Build history of the part. All positions in model axes, mm. Give positions to 0.01 mm unless a question says otherwise; leave off trailing zeros. Put each result on its own line as item: value. Start each with the question number.
Item 1: Drill centre lines: line 1 along Y through (x, z) = (0, -32.5); line 2 along Y through (x, z) = (0, -44.8); line 3 along X through (y, z) = (0, -43). Where is each one in solid material? Low to high.
Item 2: Slice it at A-A, the plane x = 0. Give the number of separate pieces and of enclosed holes in the cut face, plus the area to 3 significant figures.
Item 3: Flat gauge pins, fed straight in: pin 1 Ø2.5 at (x, z) = (-11.5, 48.5) entering from +Y; pin 2 Ø1.8 at (x, z) = (-0.5, 59.5) entering from -Y; pin 3 Ø5 at (y, z) = (-1, 26.5) entering from -X. Where does each tip first touch, or does it go through?
```python
from build123d import *

# Parameters (mm, degrees)
F3_DEPTH = 5
F5_DEPTH = 15
F6_W     = 2
F6_H     = 3
F7_DEPTH = 20.5
F8_W     = 3
F8_H     = 1
F9_DEPTH = 17.5068136575
F10_R    = 0.3
F11_R    = 0.1
F12_R    = 0.1
F13_R    = 3


with BuildPart() as f2:
    # F1 (on Front) → F2 (revolve)
    with BuildSketch(Plane.XZ):
        with BuildLine():
            Line((-2, 62), (-10, 62))
            add(Edge.make_bspline(
                [(-10, 62), (-11.8174263966, 57.1809415466), (-15.8594861297, 46.4373198499), (-18.6273544316, 24.5459471202), (-15.0414654734, -19.3469968059), (-5.4834802074, -38.7438846901), (-1.25, -47.0509425635)],
                knots=[0, 0, 0, 0, 0.1886807773, 0.4119593541, 0.7294893705, 0.9757699691, 0.9757699691, 0.9757699691, 0.9757699691], degree=3))
            Line((-1.25, -47.0509425635), (-1.25, -43.0509425635))
            Line((-1.25, -43.0509425635), (-1.75, -43.0509425635))
            Line((-1.75, -43.0509425635), (-1.75, -17))
            Line((-1.75, -17), (0, -17))
            Line((0, -17), (0, 47))
            Line((0, 47), (0, 50))
            Line((0, 50), (-2, 50))
            Line((-2, 50), (-2, 62))
        make_face()
    revolve(axis=Axis((0, 0, 54.5), (0, 0, 1)))

    # F0 (on Front) → F3 (cut, symmetric)
    with BuildSketch(Plane.XZ):
        Polygon((-10.75, -17), (10.75, -17), (10.75, 47), (9, 47), (9, 53), (-9, 53), (-9, 47), (-10.75, 47), align=None)
    extrude(amount=F3_DEPTH, both=True, mode=Mode.SUBTRACT)

    # F4 (on face) → F5 (cut)
    with BuildSketch(Plane.XY.offset(62)):
        Polygon((1.1547005384, -2), (2.3094010768, 0), (1.1547005384, 2), (-1.1547005384, 2), (-2.3094010768, 0), (-1.1547005384, -2), align=None)
    extrude(amount=-F5_DEPTH, mode=Mode.SUBTRACT)

    # F6 (on Right) → F7 (cut, symmetric)
    with BuildSketch(Plane.YZ):
        with Locations((-1, 48.5)):
            Rectangle(F6_W, F6_H)
    extrude(amount=F7_DEPTH, both=True, mode=Mode.SUBTRACT)

    # F8 (on Front) → F9 (cut, through all)
    with BuildSketch(Plane.XZ):
        with Locations((0, 41.5)):
            Rectangle(F8_W, F8_H)
    extrude(amount=F9_DEPTH, mode=Mode.SUBTRACT)

    # F10
    f10_edges = [f2.edges().sort_by_distance(p)[0] for p in [
        (1.25, 0, -47.050943),
    ]]
    fillet(f10_edges, radius=F10_R)

    # F11
    f11_edges = [f2.edges().sort_by_distance(p)[0] for p in [
        (1.25, 0, -43.050943),
    ]]
    fillet(f11_edges, radius=F11_R)

    # F12
    f12_edges = [f2.edges().sort_by_distance(p)[0] for p in [
        (1.75, 0, -43.050943),
    ]]
    fillet(f12_edges, radius=F12_R)

    # F13
    f13_edges = [f2.edges().sort_by_distance(p)[0] for p in [
        (10, 0, 62),
    ]]
    fillet(f13_edges, radius=F13_R)


solid = f2.part
```
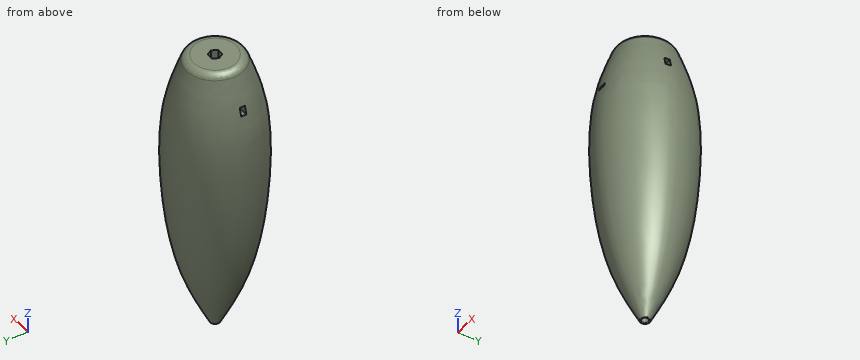
Values follow:
1. line 1: -8.11 to -1.75, 1.75 to 8.11
1. line 2: -2.39 to -1.25, 1.25 to 2.39
1. line 3: -3.29 to -1.74, 1.74 to 3.29
2. separate pieces: 3
2. enclosed holes: 0
2. area: 2,090 mm2
3. pin 1: y = 10.49
3. pin 2: y = -11.26
3. pin 3: x = -17.5
